CAD build for the part. Positions are in the model's coordinates, mm. Give positions to 0.01 mm unless a question says otherwise; leave off trailing zeros. Write each loop counter-clockwise with the first axis right and the second up, starting at its lowest first coordinate (ties: lowest second). Pieces come first, ordered by that corner, then holes. Notation, with made-up numbers: (-18.75, -7) - (13.25, -7) arc R18 cw to (13.25, 18) - close; hole circle Ø10 at (54, 30.5). An arc over 180 degrees is marked (long way). Answer as a JSON object with one key per item and string values.
from build123d import *

# Parameters (mm, degrees)
SKETCH1_W           = 90
SKETCH1_H           = 14.5
SKETCH1_R           = 2.5
SKETCH1_H_2         = 30
BOSS_EXTRUDE1_DEPTH = 3


with BuildPart() as part:
    # Sketch1 → Boss-Extrude1 (new body)
    # profile 1 of 2: a face of its own
    with BuildSketch(Plane.XY):
        with Locations((45, 7.25)):
            Rectangle(SKETCH1_W, SKETCH1_H)
        with Locations((5, 4.5)):
            Circle(SKETCH1_R, mode=Mode.SUBTRACT)
        with Locations((25, 4.5)):
            Circle(SKETCH1_R, mode=Mode.SUBTRACT)
        with Locations((45, 4.5)):
            Circle(SKETCH1_R, mode=Mode.SUBTRACT)
        with Locations((65, 4.5)):
            Circle(SKETCH1_R, mode=Mode.SUBTRACT)
        with Locations((85, 4.5)):
            Circle(SKETCH1_R, mode=Mode.SUBTRACT)
    # profile 2 of 2: a face of its own
    with BuildSketch(Plane.XY):
        with Locations((45, 29.5)):
            Rectangle(SKETCH1_W, SKETCH1_H_2)
        with Locations((5, 34.5)):
            Circle(SKETCH1_R, mode=Mode.SUBTRACT)
        with Locations((25, 34.5)):
            Circle(SKETCH1_R, mode=Mode.SUBTRACT)
        with Locations((45, 34.5)):
            Circle(SKETCH1_R, mode=Mode.SUBTRACT)
        with Locations((65, 34.5)):
            Circle(SKETCH1_R, mode=Mode.SUBTRACT)
        with Locations((85, 34.5)):
            Circle(SKETCH1_R, mode=Mode.SUBTRACT)
    extrude(amount=BOSS_EXTRUDE1_DEPTH)


solid = part.part
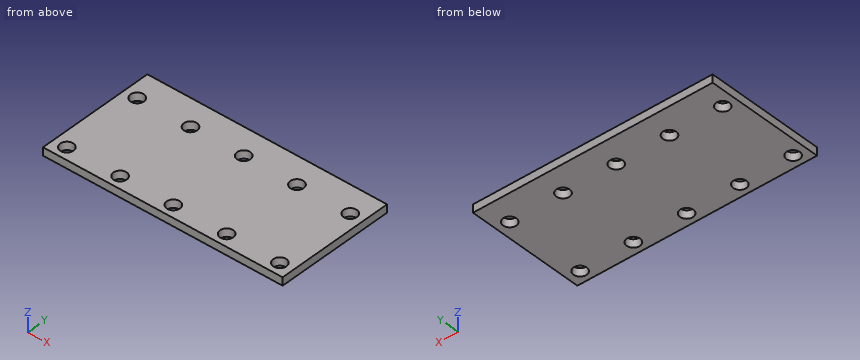
(1) Probe L1, parallel to Y at x = 5, z = 1.2; L2, parallel to X at y = 34, z = 2.3. List the from-to ranges inside material, lowest first. Write a range as [from, to].
Answer key:
{"L1": "y = [0, 2], [7, 32], [37, 44.5]", "L2": "x = [0, 2.55], [7.45, 22.55], [27.45, 42.55], [47.45, 62.55], [67.45, 82.55], [87.45, 90]"}
(2) Saw through at B-B, the plane y = 34.5. Give the cut face in (x, z).
Answer key:
{"outline": "(0, 0) - (2.5, 0) - (2.5, 3) - (0, 3) - close; (7.5, 0) - (22.5, 0) - (22.5, 3) - (7.5, 3) - close; (27.5, 0) - (42.5, 0) - (42.5, 3) - (27.5, 3) - close; (47.5, 0) - (62.5, 0) - (62.5, 3) - (47.5, 3) - close; (67.5, 0) - (82.5, 0) - (82.5, 3) - (67.5, 3) - close; (87.5, 0) - (90, 0) - (90, 3) - (87.5, 3) - close"}
(3) Saw through at A-A, the plane x = 85. Give the cut face in (y, z), and give its area (4 significant figures).
Answer key:
{"outline": "(0, 0) - (2, 0) - (2, 3) - (0, 3) - close; (7, 0) - (32, 0) - (32, 3) - (7, 3) - close; (37, 0) - (44.5, 0) - (44.5, 3) - (37, 3) - close", "area": "103.5 mm²"}
(4) Saw through at D-D, the plane y = 5.5. Give the cut face in (x, z).
Answer key:
{"outline": "(0, 0) - (2.71, 0) - (2.71, 3) - (0, 3) - close; (7.29, 0) - (22.71, 0) - (22.71, 3) - (7.29, 3) - close; (27.29, 0) - (42.71, 0) - (42.71, 3) - (27.29, 3) - close; (47.29, 0) - (62.71, 0) - (62.71, 3) - (47.29, 3) - close; (67.29, 0) - (82.71, 0) - (82.71, 3) - (67.29, 3) - close; (87.29, 0) - (90, 0) - (90, 3) - (87.29, 3) - close"}
(5) Saw through at C-C, the plane z = 1.7. State how many separate pieces and enclosed holes the cut face has, and give its area (3 significant figures).
Answer key:
{"separate pieces": "1", "enclosed holes": "10", "area": "3,810 mm²"}
(6) Flat gauge pin, fed straight in: P1, Ø3, axis at x = 5, y = 34.5, coming from the -Z side. Where does the tip first touch, or does it go through?
Answer key:
{"P1": "passes through"}
